Read the model definition and answer for the solid it produces. Units are mm, in the model's axes. Face numbers are marked on the shaded views. A direction names the side the tool comes from. Coordinates: 2 decimals unless noted, no trailing zeros.
from build123d import *

# Parameters (mm, degrees)
F0_R      = 24.4192579829
F1_DEPTH  = 20
F5_DEPTH  = 0.8
F6_R      = 3.0326267801
F7_DEPTH  = 40
F8_R      = 2
F9_SIZE   = 1
F10_DEPTH = 25
F10_TAPER = -10


with BuildPart() as f1:
    # F0 (on Top) → F1 (new body)
    with BuildSketch(Plane.XY):
        Circle(F0_R)
    extrude(amount=F1_DEPTH)

    # F4 (on offset) → F5 (join)
    with BuildSketch(Plane.XY.offset(2.5)):
        with BuildLine():
            ThreePointArc((4.3520725579, 24.0283088229), (8.3888871456, 22.9330925279), (12.179572853, 21.1650222196))
            ThreePointArc((12.179572853, 21.1650222196), (9.2528939627, 25.2950683106), (4.3520725579, 24.0283088229))
        make_face()
    extrude(amount=F5_DEPTH)

    # F6 (on Front) → F7 (join)
    with BuildSketch(Plane.XZ):
        with Locations((0, 9.6028381959)):
            Circle(F6_R)
    extrude(amount=F7_DEPTH)

    # F8
    f8_edges = [f1.edges().sort_by_distance(p)[0] for p in [
        (-24.419258, 0, 20),
        (-3.032627, -24.230215, 9.602838),
    ]]
    fillet(f8_edges, radius=F8_R)

    # F9
    f9_edges = [f1.edges().sort_by_distance(p)[0] for p in [
        (-3.032627, -40, 9.602838),
    ]]
    chamfer(f9_edges, length=F9_SIZE)

    # F2 (on Top) → F10 (join)
    with BuildSketch(Plane.XY):
        with BuildLine():
            ThreePointArc((4.3520725579, 24.0283088229), (-18.7426591361, -15.6528875592), (24.4192579829, 0))
            ThreePointArc((24.4192579829, 0), (21.1390195143, 12.2246478235), (12.179572853, 21.1650222196))
            ThreePointArc((12.179572853, 21.1650222196), (8.3888871456, 22.9330925279), (4.3520725579, 24.0283088229))
        make_face()
    extrude(amount=-F10_DEPTH, taper=F10_TAPER)


solid = f1.part
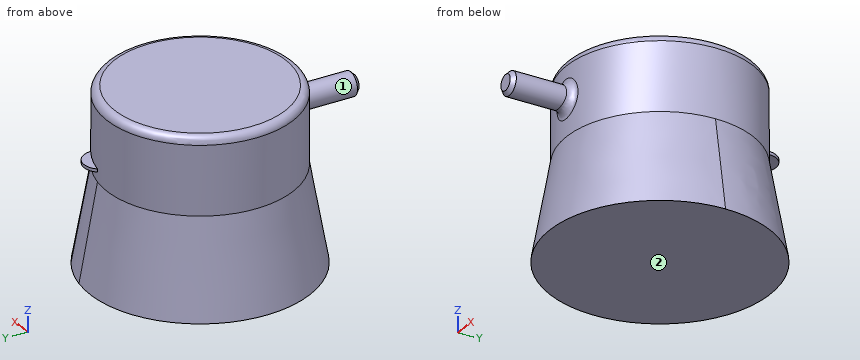
Item 1: Which of the six approach directions +Z, -Z, +X, -X, +Y, -Y give full straight-line access (tool end or side, diameter ignored) to the marked faces 1 and 2?
Numbers:
face 1: -Y
face 2: -Z, +X, -X, +Y, -Y
Item 2: Given pin 1 (4 mm diameter, centred on x = -4, z = -8, fed in from +Y); pin 2 (10 mm diameter, centred on y = 5, z = -3, fed in from -X); pin 3 (3 mm diameter, centred on x = -16, z = 7.5, fed in from -Y), each flat-ended and moving along its own axis, determine where each tip first touches the part or whether it passes through.
Numbers:
pin 1: stops at y = 25.96
pin 2: stops at x = -25.59
pin 3: stops at y = -19.65
Item 3: Find the intervals of material crossed by line 1 along Y through (x, z) = (23, -14); line 2 along Y through (x, z) = (7, 5); line 3 along X through (y, z) = (-25, 8.5), in increasing order.
Numbers:
line 1: y = -13.93 to 13.93
line 2: y = -23.39 to 23.39
line 3: x = -3.1 to 3.1
